Could you check a few things on this drawing? It's one solid part, dimensions in mm from its lowest x, y, z. Round coordinates to 2 decimals unless told otherwise and drop trailing zeros. Loops run counter-clockwise (first coordinate to the right, second up) from the corner with the lowest first, then second, coordinate; pieces in that order, holes last.
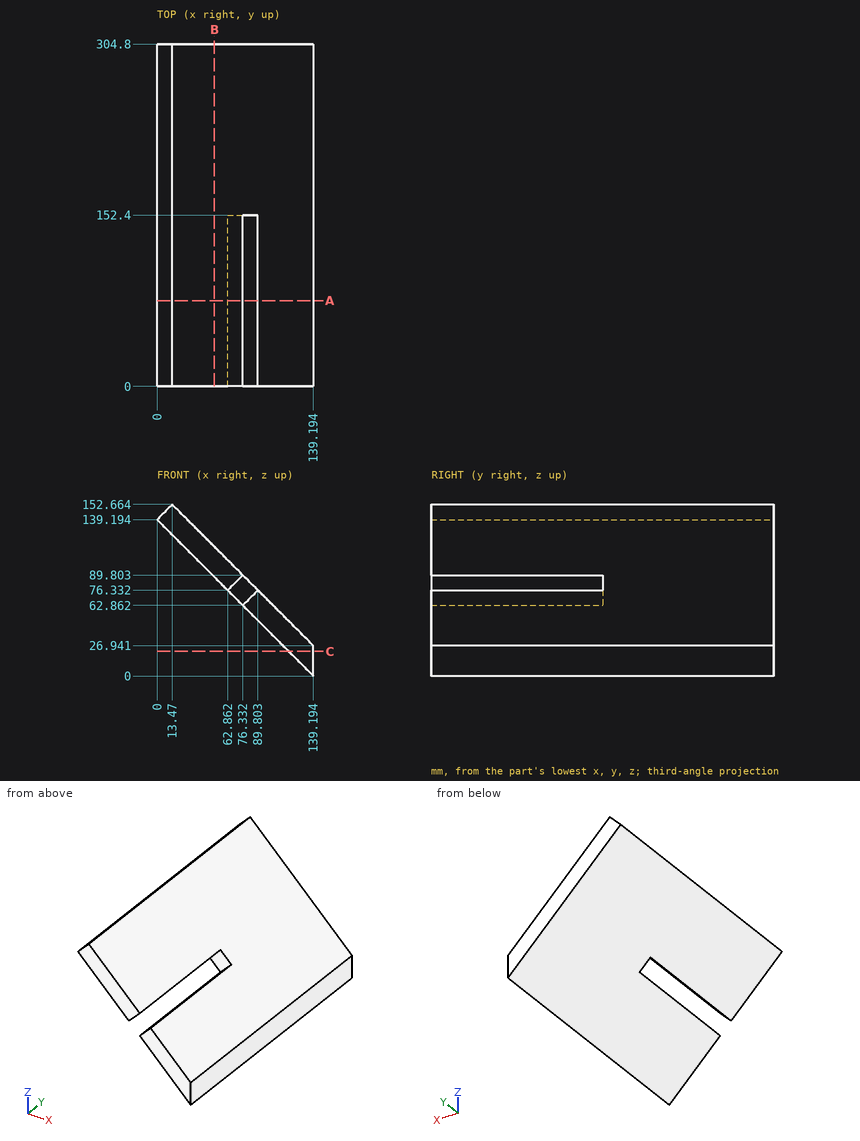
(1) For pin 1 (1 mm diameter, centred on x = 91.5, y = 105, fed in from +Z) (1 decimal); pin 2 (8 mm diameter, centred on x = 53.5, y = 142, fed in from -Z) (1 decimal); pin 3 (5 mm diameter, centred on y = 263.5, z = 135.5, fed in from +X) (1 decimal), each with a flat end and sliding along its axis, tell me the tip position at first contact or that it passes through.
(2) Suppose I cut it at B-B (x = 51). Write out the boundary of the cut face in (y, z) (1 decimal).
(3) Suppose I cut it at A-A (y = 76.5). Write out the boundary of the cut face in (x, z) (1 decimal), then the cut area to 3 significant figures.
(4) Suppose I cut it at C-C (z = 22). Write out the boundary of the cut face in (x, y), then the cut area to 3 significant figures.
(5) If I drill on line 1 (Y direction, x = 85, z = 73); line 2 (X direction, y = 101, z = 138) (1 decimal); line 3 (X direction, y = 172.5, z = 59.5) (1 decimal), over which ranges is the centre line in solid material (lowest first)?
Check result:
1. pin 1: stops at z = 75.1
1. pin 2: stops at z = 81.7
1. pin 3: stops at x = 33.1
2. outline: (0, 88.2) - (304.8, 88.2) - (304.8, 115.1) - (0, 115.1) - close
3. outline: (0, 139.2) - (62.9, 76.3) - (76.3, 89.8) - (13.5, 152.7) - close; (76.3, 62.9) - (139.2, 0) - (139.2, 26.9) - (89.8, 76.3) - close
3. area: 3,210 mm2
4. outline: (117.19, 0) - (139.19, 0) - (139.19, 304.8) - (117.19, 304.8) - close
4. area: 6,710 mm2
5. line 1: y = 152.4 to 304.8
5. line 2: x = 1.2 to 28.1
5. line 3: x = 79.7 to 106.6
